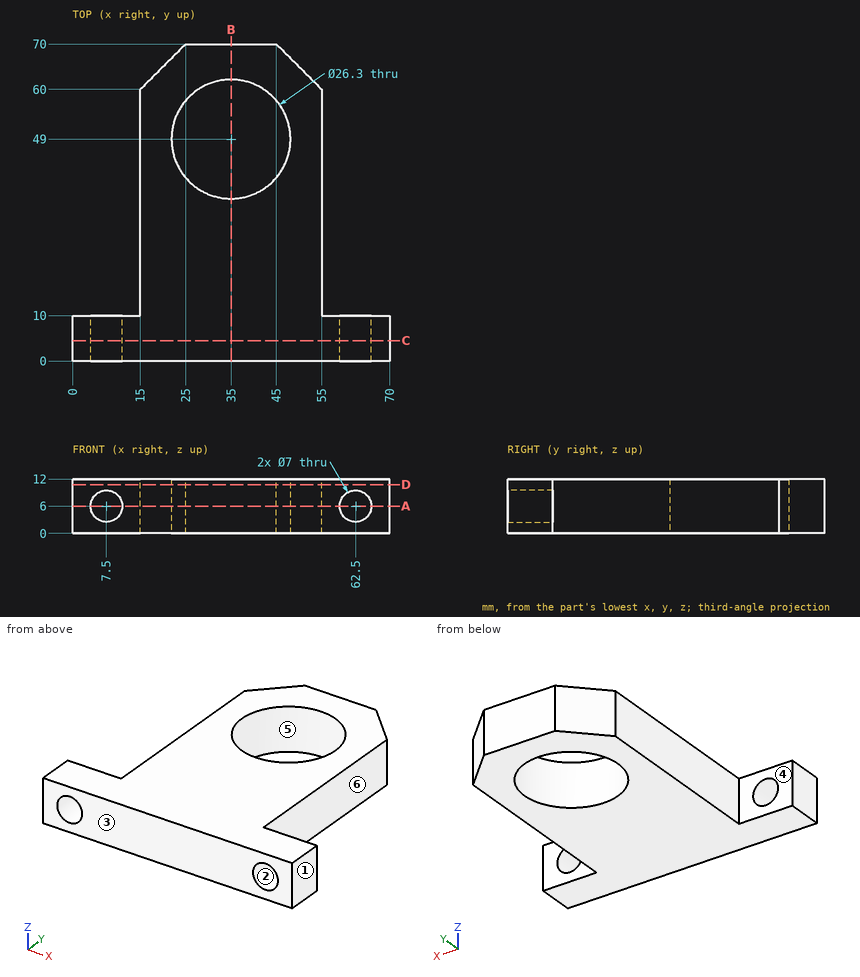
Job drawing, mm, ordinate dimensions from the low corner. One solid piece. A direction names the side the tool comes from. Round coordinates to 2 decimals unless told otherwise and drop trailing zeros. Loops run counter-clockwise (first coordinate to the right, second up) from the corner with the lowest first, then second, coordinate; pieces in that order, holes last.
(1) Wall check: line 1 along X through (y, z) = (7.25, 6); line 2 along Y through (x, z) = (35, 7); line 3 along Y through (x, z) = (59, 11.5). Give the ranges that are in metal, low to high.
(2) Drop flat-ended pins along their axis: pin 1 (3.5 mm diameter, centred on y = 32, z = 5, fed in from -X); pin 2 (5 mm diameter, centred on y = 53.5, z = 5, fed in from +X); pin 3 (2 mm diameter, centred on x = 25.5, y = 11, fed in from -Z); pin 4 (23.5 mm diameter, centred on x = 35, y = 49, fed in from +Z). Give the stop position or say it passes through.
(3) Cut at C-C (y = 4.5). Give the cut face in (x, z).
(4) Cut at A-A (z = 6). Give the cut face in (x, y), plus the area to 3 significant figures.
(5) Which spindle directions (+Z, -Z, +X, -X, +Y, -Y) get a long thin tool onto all of the face, cutting with end or side? Do the marked faces 4, 5 and 6. Say none if no direction does.
(6) Cut at B-B (x = 35). Give the cut face in (y, z).
(7) Two-plate mould, pull along X, no slides. Class the marked faces 1, 2 and 3: +X half, -X half, draft (parallel to the pull), parting line (faces both ways), or undercut.
(8) Cut at D-D (z = 10.75). Give the cut face in (x, y).
Findings below:
1. line 1: x = 0 to 4, 11 to 59, 66 to 70
1. line 2: y = 0 to 35.85, 62.15 to 70
1. line 3: y = 0 to 10
2. pin 1: stops at x = 15
2. pin 2: stops at x = 55
2. pin 3: stops at z = 0
2. pin 4: passes through
3. outline: (0, 0) - (70, 0) - (70, 12) - (0, 12) - close; hole circle Ø7 at (7.5, 6); hole circle Ø7 at (62.5, 6)
4. outline: (0, 0) - (4, 0) - (4, 10) - (0, 10) - close; (11, 0) - (59, 0) - (59, 10) - (55, 10) - (55, 60) - (45, 70) - (25, 70) - (15, 60) - (15, 10) - (11, 10) - close; (66, 0) - (70, 0) - (70, 10) - (66, 10) - close; hole circle Ø26.3 at (35, 49)
4. area: 2,320 mm2
5. face 4: +Z, -Z, -X, +Y
5. face 5: +Z, -Z
5. face 6: +Z, -Z, +X, +Y
6. outline: (0, 0) - (35.85, 0) - (35.85, 12) - (0, 12) - close; (62.15, 0) - (70, 0) - (70, 12) - (62.15, 12) - close
7. face 1: +X half
7. face 2: undercut
7. face 3: draft
8. outline: (0, 0) - (70, 0) - (70, 10) - (55, 10) - (55, 60) - (45, 70) - (25, 70) - (15, 60) - (15, 10) - (0, 10) - close; hole circle Ø26.3 at (35, 49)
